Source: CAD feature listing. Evaluate the final solid. Frame: model axes, mm. A direction names the side the tool comes from. Give positions to 0.01 mm unless a question says otherwise; leave off trailing zeros. Loops run counter-clockwise (first coordinate to the right, second up) from the corner with the lowest first, then second, coordinate; pieces in that order, holes last. Notation, with made-up numbers: (4, 45) -> (32, 45) arc R17 cw to (32, 62) -> close; hole circle Ø9 at (2.25, 16). An arc over 180 degrees is marked (long way). Return JSON: item names as keys, results as strings. Group by question number.
(1) Cut plane B-B on z = -33.1. Return loops of the section in (x, y).
(2) Draft query along X for faces 1 (the face through (3.189, 3.451, -74.932)), 2 (the face through (-56.057, 4.313, -38.835)), 3 (the face through (-1, 0, -55)). Return one class per face: released by +X, released by -X, zero draft, split by the parting line, or undercut.
(3) Cut plane C-C on y = 5. Give the number of separate pieces and of enclosed holes in the cut face, then the cut area to 3 significant figures.
(4) Ray query, line 1 (X direction, y = 5.5, z = -30); line 2 (X direction, y = 1.1, z = -33.1); line 3 (Z direction, x = -22, y = 6.25). Return the intervals inside material, ascending. Write a range as from..to.
(5) Access query for faces 4 (the face through (54.6, 4.3, -38.3)), 5 (the face through (-1, 3, -8)), 6 (the face through (-1, 7, -55)). Directions: +Z, -Z, +X, -X, +Y, -Y. A direction counts if a zero-diameter tool reaches every point of the face in a straight line with its end or side. Return the directions, or none.
(6) Cut plane A-A on x = 0. Return loops of the section in (y, z) (3 decimals).
(7) Pin query (flat end, axial travel): pin 1 (13 mm diameter, centred on x = 21.5, z = -62, fed in from +Y); pin 2 (9.5 mm diameter, centred on x = 57.5, z = -33, fed in from +Y); pin 3 (2 mm diameter, centred on x = 10.5, y = 4, fed in from -Z). Return the tip coordinate at first contact, or that it passes through.
(8) Cut plane D-D on x = -31.5. Return loops of the section in (y, z).
```python
from build123d import *

# Parameters (mm, degrees)
SKETCH1_R           = 75
BOSS_EXTRUDE1_DEPTH = 7
SKETCH2_R           = 5.875
CUT_EXTRUDE1_DEPTH  = 5.45
SKETCH3_R           = 4
CUT_EXTRUDE2_DEPTH  = 2.55
CIRPATTERN1_COUNT   = 18
FILLET1_R           = 3


with BuildPart() as part:
    # Sketch1 → Boss-Extrude1 (new body)
    with BuildSketch(Plane(origin=(0, 0, 0), x_dir=(1, 0, 0), z_dir=(0, 1, 0))):
        Circle(SKETCH1_R)
        with BuildLine():
            Line((-51.709821359, 8), (51.709821359, 8))
            ThreePointArc((51.709821359, 8), (0, 52.325), (-51.709821359, 8))
        make_face(mode=Mode.SUBTRACT)
    extrude(amount=BOSS_EXTRUDE1_DEPTH)

    # Sketch2 → Cut-Extrude1 (cut)
    with BuildSketch(Plane(origin=(0, 7, 0), x_dir=(1, 0, 0), z_dir=(0, 1, 0))):
        with Locations((0, 66.2)):
            Circle(SKETCH2_R)
    cut_extrude1 = extrude(amount=-CUT_EXTRUDE1_DEPTH, mode=Mode.SUBTRACT)

    # Sketch3 → Cut-Extrude2 (cut, through all)
    with BuildSketch(Plane(origin=(0, 1.55, 0), x_dir=(1, 0, 0), z_dir=(0, 1, 0))):
        with Locations((0, 66.2)):
            Circle(SKETCH3_R)
    cut_extrude2 = extrude(amount=-CUT_EXTRUDE2_DEPTH, mode=Mode.SUBTRACT)

    # CirPattern1: Cut-Extrude1, Cut-Extrude2 ×18 about axis
    cirpattern1_axis = Axis((0, 0, 0), (0, 1, 0))
    for i in range(1, CIRPATTERN1_COUNT):
        add(cut_extrude1.rotate(cirpattern1_axis, i * 360 / CIRPATTERN1_COUNT), mode=Mode.SUBTRACT)
        add(cut_extrude2.rotate(cirpattern1_axis, i * 360 / CIRPATTERN1_COUNT), mode=Mode.SUBTRACT)

    # Split1
    split(bisect_by=Plane.XY, keep=Keep.BOTTOM)

    # Fillet1
    fillet1_edges = [part.edges().sort_by_distance(p)[0] for p in [
        (51.709821359, 3.5, -8),
        (-51.709821359, 3.5, -8),
        (-75, 3.5, 0),
    ]]
    fillet(fillet1_edges, radius=FILLET1_R)


solid = part.part
```
Answers:
{
 "1": {"outline": "(-67.3, 0) -> (-61.33, 0) -> (-61.33, 1.55) -> (-63.21, 1.55) -> (-63.21, 7) -> (-67.3, 7) -> close; (-53.33, 0) -> (-40.53, 0) -> (-40.53, 7) -> (-51.46, 7) -> (-51.46, 1.55) -> (-53.33, 1.55) -> close; (40.53, 0) -> (53.33, 0) -> (53.33, 1.55) -> (51.46, 1.55) -> (51.46, 7) -> (40.53, 7) -> close; (61.33, 0) -> (67.3, 0) -> (67.3, 7) -> (63.21, 7) -> (63.21, 1.55) -> (61.33, 1.55) -> close"},
 "2": {"face 1": "split by the parting line", "face 2": "undercut", "face 3": "zero draft"},
 "3": {"separate pieces": "1", "enclosed holes": "10", "area": "4,400 mm²"},
 "4": {"line 1": "-68.74..-62.32, -52.34..-42.87, 42.87..52.34, 62.32..68.74", "line 2": "-67.3..-61.33, -53.33..-40.53, 40.53..53.33, 61.33..67.3", "line 3": "-71.7..-68.05, -56.37..-47.48, -8..0"},
 "5": {"face 4": "+Y", "face 5": "+Y, -Y", "face 6": "+Z, -Z, +X, -X, +Y"},
 "6": {"outline": "(0, -75) -> (7, -75) -> (7, -72.075) -> (1.55, -72.075) -> (1.55, -70.2) -> (0, -70.2) -> close; (0, -62.2) -> (1.55, -62.2) -> (1.55, -60.325) -> (7, -60.325) -> (7, -52.325) -> (0, -52.325) -> close; (0, -8) -> (7, -8) -> (7, 0) -> (0, 0) -> close"},
 "7": {"pin 1": "y = 7", "pin 2": "y = 1.55", "pin 3": "z = -74.4"},
 "8": {"outline": "(0, -68.06) -> (7, -68.06) -> (7, -41.78) -> (0, -41.78) -> close; (0, -8) -> (7, -8) -> (7, 0) -> (0, 0) -> close"}
}
